```python
from build123d import *

# Parameters (mm, degrees)
SKETCH1_W           = 270
SKETCH1_H           = 64
BOSS_EXTRUDE1_DEPTH = 6.88
SKETCH2_W           = 20
SKETCH2_H           = 27
SKETCH2_W_2         = 152
SKETCH2_H_2         = 16
CUT_EXTRUDE1_DEPTH  = 139.911246485
SKETCH3_R           = 2.25
CUT_EXTRUDE2_DEPTH  = 139.911246485
BOSS_EXTRUDE2_DEPTH = 6.88
SKETCH5_W           = 2.085
SKETCH5_H           = 5
SKETCH5_W_2         = 3.55
SKETCH5_H_2         = 11
CUT_EXTRUDE3_DEPTH  = 144.113012686
SKETCH7_W           = 14.25
SKETCH7_H           = 26.5
SKETCH7_W_2         = 19
SKETCH7_H_2         = 10
CUT_EXTRUDE4_DEPTH  = 144.113012686
SKETCH8_W           = 52
SKETCH8_H           = 8
BOSS_EXTRUDE4_DEPTH = 6.88
CUT_EXTRUDE5_DEPTH  = 144.113012686
FILLET2_R           = 0.5
CUT_EXTRUDE6_DEPTH  = 144.113012686
FILLET1_R           = 2.5
FILLET3_R           = 15


with BuildPart() as part:
    # Sketch1 → Boss-Extrude1 (new body)
    with BuildSketch(Plane.XY):
        Rectangle(SKETCH1_W, SKETCH1_H)
    extrude(amount=BOSS_EXTRUDE1_DEPTH)

    # Sketch2 → Cut-Extrude1 (cut, through all)
    with BuildSketch(Plane.XY.offset(6.88)):
        with Locations((65, 0.5)):
            Rectangle(SKETCH2_W, SKETCH2_H)
        with Locations((-29, -24)):
            Rectangle(SKETCH2_W_2, SKETCH2_H_2)
    extrude(amount=-CUT_EXTRUDE1_DEPTH, mode=Mode.SUBTRACT)

    # Sketch3 → Cut-Extrude2 (cut, through all)
    with BuildSketch(Plane.XY.offset(6.88)):
        with Locations((-102.5, -11.5)):
            Circle(SKETCH3_R)
        with Locations((47.5, -11.5)):
            Circle(SKETCH3_R)
    extrude(amount=-CUT_EXTRUDE2_DEPTH, mode=Mode.SUBTRACT)

    # Sketch4 → Boss-Extrude2 (add)
    with BuildSketch(Plane.XY.offset(6.88)):
        Polygon((47, -32), (67, -32), (67, -39), (75, -39), (75, -47), (47, -47), align=None)
    extrude(amount=-BOSS_EXTRUDE2_DEPTH)

    # Sketch5 → Cut-Extrude3 (cut, through all)
    with BuildSketch(Plane.XY.offset(6.88)):
        with Locations((-117.1825, -18.5)):
            Rectangle(SKETCH5_W, SKETCH5_H)
        with Locations((-120, -18.5)):
            Rectangle(SKETCH5_W_2, SKETCH5_H)
        with Locations((-120, -13.5)):
            Rectangle(SKETCH5_W_2, SKETCH5_H)
        with Locations((-122.8175, -18.5)):
            Rectangle(SKETCH5_W, SKETCH5_H)
        with Locations((-120, -26.5)):
            Rectangle(SKETCH5_W_2, SKETCH5_H_2)
    extrude(amount=-CUT_EXTRUDE3_DEPTH, mode=Mode.SUBTRACT)

    # Sketch7 → Cut-Extrude4 (cut, through all)
    with BuildSketch(Plane(origin=(0, 0, 0), x_dir=(-1, 0, 0), z_dir=(0, 0, -1))):
        with Locations((22.375, 0.25)):
            Rectangle(SKETCH7_W, SKETCH7_H)
        with Locations((48.5, -8)):
            Rectangle(SKETCH7_W_2, SKETCH7_H_2)
    extrude(amount=-CUT_EXTRUDE4_DEPTH, mode=Mode.SUBTRACT)

    # Sketch8 → Boss-Extrude4 (add)
    with BuildSketch(Plane(origin=(0, 0, 0), x_dir=(-1, 0, 0), z_dir=(0, 0, -1))):
        with Locations((39.125, -17)):
            Rectangle(SKETCH8_W, SKETCH8_H)
    extrude(amount=-BOSS_EXTRUDE4_DEPTH)

    # Sketch9 → Cut-Extrude5 (cut, through all)
    with BuildSketch(Plane(origin=(0, 0, 0), x_dir=(-1, 0, 0), z_dir=(0, 0, -1))):
        with BuildLine():
            Line((-77, -32), (-127, -32))
            ThreePointArc((-127, -32), (-102, -17), (-77, -32))
        make_face()
    extrude(amount=-CUT_EXTRUDE5_DEPTH, mode=Mode.SUBTRACT)

    # Fillet2
    fillet2_edges = [part.edges().sort_by_distance(p)[0] for p in [
        (-116.14, -16, 3.44),
        (-116.14, -21, 3.44),
        (-123.86, -21, 3.44),
        (-123.86, -16, 3.44),
    ]]
    fillet(fillet2_edges, radius=FILLET2_R)

    # Sketch10 → Cut-Extrude6 (cut, through all)
    with BuildSketch(Plane.XY.offset(6.88)):
        Polygon((80, 32), (135, 15), (135, 32), align=None)
    extrude(amount=-CUT_EXTRUDE6_DEPTH, mode=Mode.SUBTRACT)

    # Fillet1
    fillet1_edges = [part.edges().sort_by_distance(p)[0] for p in [
        (55, 14, 3.44),
        (75, 14, 3.44),
        (75, -13, 3.44),
        (55, -13, 3.44),
        (-135, 32, 3.44),
        (-135, -32, 3.44),
        (47, -16, 3.44),
        (-105, -16, 3.44),
        (-105, -32, 3.44),
        (75, -47, 3.44),
        (75, -39, 3.44),
        (135, -32, 3.44),
        (-58, -13, 3.44),
        (-39, -13, 3.44),
        (-39, -3, 3.44),
        (-58, -3, 3.44),
        (-29.5, 13.5, 3.44),
        (-15.25, 13.5, 3.44),
        (-15.25, -13, 3.44),
        (-29.5, -13, 3.44),
        (-65.125, -16, 3.44),
        (-65.125, -21, 3.44),
        (-13.125, -21, 3.44),
        (-13.125, -16, 3.44),
        (127, -32, 3.44),
        (77, -32, 3.44),
        (135, 15, 3.44),
        (80, 32, 3.44),
    ]]
    fillet(fillet1_edges, radius=FILLET1_R - 0.0001)  # a hair under: the kernel refuses the full size

    # Fillet3
    fillet3_edges = [part.edges().sort_by_distance(p)[0] for p in [
        (47, -47, 3.44),
    ]]
    fillet(fillet3_edges, radius=FILLET3_R)


solid = part.part
```
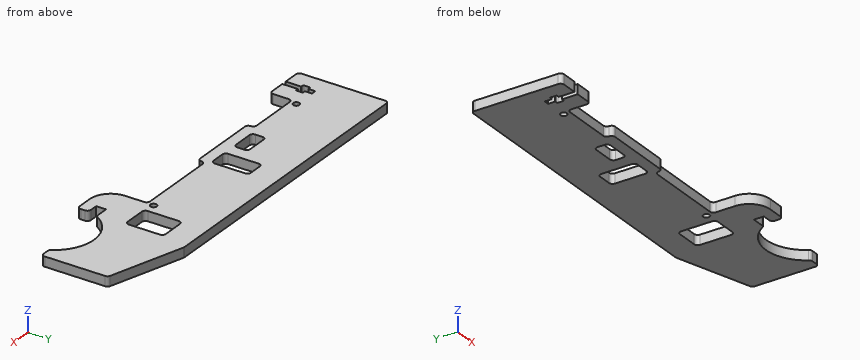
Design review of the part built by this model. Coordinates are the model's own, in mm. Round coordinates to 2 decimals unless told otherwise and drop trailing zeros. Write each loop counter-clockwise with the first axis right and the second up, starting at its lowest first coordinate (ties: lowest second). Pieces come first, ordered by that corner, then holes. Notation, with made-up numbers: (46, 20) -> (70, 20) arc R23 cw to (70, 45) -> close; hole circle Ø1 at (43, 22). An arc over 180 degrees is marked (long way). Answer in a Markdown table with one row per item.
Q1. Take a section at B-B, the plane x = -20.5. State the section outline as (y, z) points, then the cut area to 3 significant figures.
The answers:
| item | result |
|---|---|
| outline | (-21, 0) -> (-13, 0) -> (-13, 6.88) -> (-21, 6.88) -> close; (13.5, 0) -> (32, 0) -> (32, 6.88) -> (13.5, 6.88) -> close |
| area | 182 mm² |
Q2. Take a section at A-A, the plane y = 5. State the section outline as (x, z) points.
The answers:
| item | result |
|---|---|
| outline | (-135, 0) -> (-29.5, 0) -> (-29.5, 6.88) -> (-135, 6.88) -> close; (-15.25, 0) -> (55, 0) -> (55, 6.88) -> (-15.25, 6.88) -> close; (75, 0) -> (135, 0) -> (135, 6.88) -> (75, 6.88) -> close |
Q3. Take a section at D-D, the plane z = 2. Count the separate pieces of the cut face and the enclosed holes in it, then the cut area to 3 significant figures.
The answers:
| item | result |
|---|---|
| separate pieces | 1 |
| enclosed holes | 5 |
| area | 13,200 mm² |
Q4. Clearance check with flat-ended pins moving along their axes: pin 1 Ø3 at (x, z) = (57.5, 1.5) entering from -Y; pin 2 Ø2 at (x, z) = (-21.5, 4) entering from -Y; pin 3 Ø7 at (x, y) = (47.5, -11.5) entering from +Z; pin 4 Ø2 at (y, z) = (-35, 2.5) entering from +X. State where each tip first meets the part, or that it passes through.
The answers:
| item | result |
|---|---|
| pin 1 | y = -46.7 |
| pin 2 | y = -21 |
| pin 3 | z = 6.88 |
| pin 4 | x = 67 |
Q5. To check wall thickness, follow L1, parallel to Y at x = -41, z = 1; L2, parallel to X at y = -2.5, z = 1.75; L3, parallel to Y at x = -102.5, z = 3.25. State the ranges of each line that lie inside material, in increasing order. Write a range as [from, to].
The answers:
| item | result |
|---|---|
| L1 | [-21, -12.95], [-3.05, 32] |
| L2 | [-135, -29.5], [-15.25, 55], [75, 135] |
| L3 | [-16, -13.75], [-9.25, 32] |
Q6. Take a section at C-C, the plane y = -24. State the section outline as (x, z) points (3 decimals), then the cut area to 3 significant figures.
The answers:
| item | result |
|---|---|
| outline | (-135, 0) -> (-121.775, 0) -> (-121.775, 6.88) -> (-135, 6.88) -> close; (-118.225, 0) -> (-105, 0) -> (-105, 6.88) -> (-118.225, 6.88) -> close; (47, 0) -> (83.354, 0) -> (83.354, 6.88) -> (47, 6.88) -> close; (120.646, 0) -> (135, 0) -> (135, 6.88) -> (120.646, 6.88) -> close |
| area | 531 mm² |
